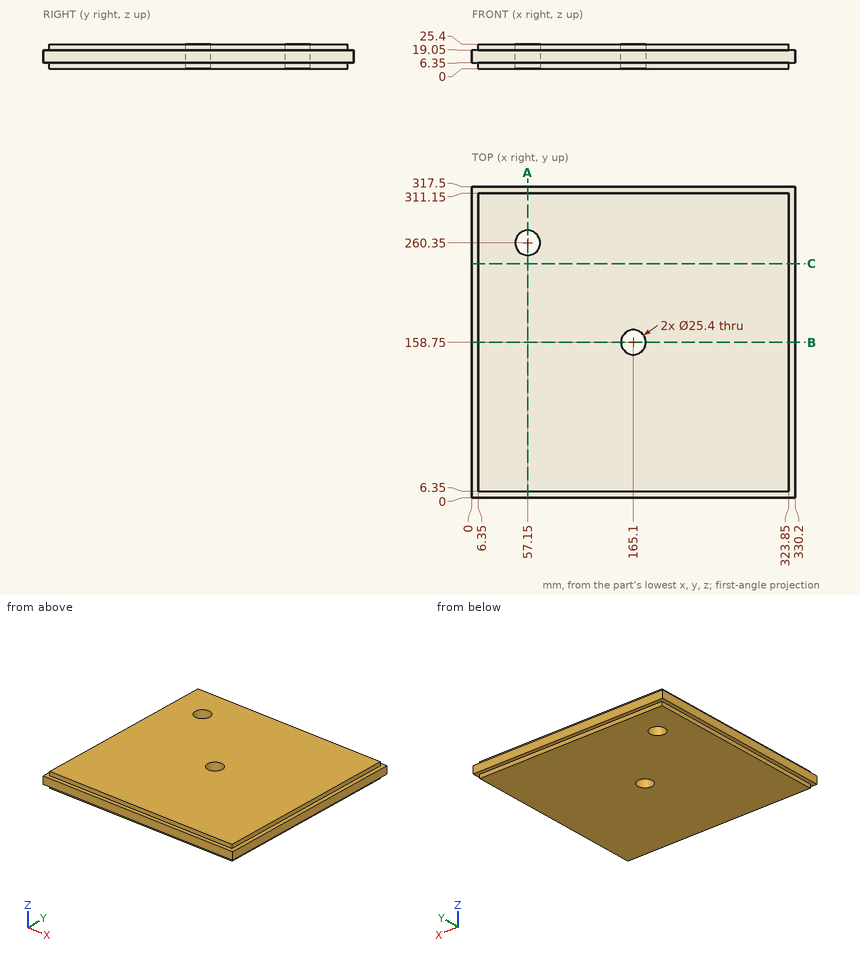
Print and shaded views of the part. All mm, measured from the part's lowest x, y and z. Coordinates: 2 decimals unless noted, no trailing zeros. Order: outer loops, then holes, each group sorted by start corner. A loop starts at its lowest first (then second) coordinate and runs counter-clockwise, first axis right, second up. Notation, with made-up numbers: (38, 13.5) - (67, 13.5) arc R10 ccw to (67, 29.5) - close; hole circle Ø9 at (33.5, 47). An arc over 180 degrees is marked (long way). Return JSON: item names as keys, results as strings. Group by question number.
Item 1: Cut at A-A (x = 57.15). List the corners of the cut face in (y, z), plus the area to 3 significant figures.
Item 2: Cut at B-B (y = 158.75). List the corners of the cut face in (x, z), plus the area to 3 significant figures.
Item 3: Pin check, flat tips, straight feed: pin 1 (5 mm diameter, centred on y = 166, z = 23.5, fed in from +X); pin 2 (5 mm diameter, centred on y = 129, z = 23, fed in from -X); pin 3 (1.9 mm diameter, centred on x = 138, z = 3.5, fed in from +Y). Stop position of each tip, or through.
Item 4: Cut at C-C (y = 239). List the corners of the cut face in (x, z), plus the area to 3 significant figures.
Item 5: Drill centre lines: probe 1 along Y at (x, z) = (165.1, 19.5); probe 2 along X at (y, z) = (260.35, 12.5); probe 3 along Y at (x, z) = (165.1, 11.25). Where is each one in solid material? Low to high. Write a range as from..to.
Check values:
{
 "1": {"outline": "(0, 6.35) - (6.35, 6.35) - (6.35, 0) - (247.65, 0) - (247.65, 25.4) - (6.35, 25.4) - (6.35, 19.05) - (0, 19.05) - close; (273.05, 0) - (311.15, 0) - (311.15, 6.35) - (317.5, 6.35) - (317.5, 19.05) - (311.15, 19.05) - (311.15, 25.4) - (273.05, 25.4) - close", "area": "7,260 mm2"},
 "2": {"outline": "(0, 6.35) - (6.35, 6.35) - (6.35, 0) - (152.4, 0) - (152.4, 25.4) - (6.35, 25.4) - (6.35, 19.05) - (0, 19.05) - close; (177.8, 0) - (323.85, 0) - (323.85, 6.35) - (330.2, 6.35) - (330.2, 19.05) - (323.85, 19.05) - (323.85, 25.4) - (177.8, 25.4) - close", "area": "7,580 mm2"},
 "3": {"pin 1": "stops at x = 323.85", "pin 2": "stops at x = 6.35", "pin 3": "stops at y = 311.15"},
 "4": {"outline": "(0, 6.35) - (6.35, 6.35) - (6.35, 0) - (323.85, 0) - (323.85, 6.35) - (330.2, 6.35) - (330.2, 19.05) - (323.85, 19.05) - (323.85, 25.4) - (6.35, 25.4) - (6.35, 19.05) - (0, 19.05) - close", "area": "8,230 mm2"},
 "5": {"probe 1": "y = 6.35..146.05, 171.45..311.15", "probe 2": "x = 0..44.45, 69.85..330.2", "probe 3": "y = 0..146.05, 171.45..317.5"}
}
